Autodesk Inventor part; units mm, degrees
ref_plane "YZ Plane" through (0, 0, 0) normal (1, 0, 0) x (0, 1, 0)
ref_plane "XZ Plane" through (0, 0, 0) normal (0, 1, 0) x (-1, 0, 0)
ref_plane "XY Plane" through (0, 0, 0) normal (0, 0, 1) x (1, 0, 0)
sketch "Sketch1" plane through (0, 0, 0) normal (0, 0, 1) x (1, 0, 0)
  line L0 (0, 0) -> (0, 80)
  line L1 (0, 0) -> (25, 0)
  line L2 (25, 0) -> (25, 80)
  arc A0 (25, 80) -> (0, 80) centre (12.5, 58.3494) ccw
  dimension "d2" = 80
  dimension "d4" = 25
  dimension "d5" = 80
  dimension "d6" = 25
extrude "Extrusion1" add sketch "Sketch1" along normal blind 3
sketch "Sketch2" plane through (0, 0, 3) normal (0, 0, 1) x (1, 0, 0)
  circle A0 centre (12.5, 67.7859) radius 10
  point P0 (0, 0)
  dimension "d9" = 20
extrude "Extrusion2" cut sketch "Sketch2" against normal blind 3
sketch "Sketch3" plane through (0, 0, 0) normal (0, -1, 0) x (1, 0, 0)
  line L0 (25, 0) -> (0, 0)
  line L1 (25, 3) -> (0, 3)
  line L2 (0, 0) -> (25, 0)
  line L3 (25, 0) -> (25, 3)
  line L4 (25, 3) -> (0, 3)
  line L5 (0, 3) -> (0, 0)
extrude "Extrusion3" add sketch "Sketch3" along normal blind 50
sketch "Sketch4" plane through (0, -50, 0) normal (0, -1, 0) x (1, 0, 0)
  line L0 (0, 0) -> (0, 3)
  line L1 (25, 0) -> (25, 3)
  line L2 (0, 3) -> (25, 3)
  line L3 (25, 3) -> (25, 0)
  line L4 (25, 0) -> (0, 0)
  line L5 (0, 0) -> (0, 3)
sketch "Sketch5" plane through (0, 0, 3) normal (0, 0, 1) x (1, 0, 0)
  circle A0 centre (12.7766, 13.1416) radius 10
  point P0 (0, 0)
  dimension "d14" = 20
extrude "Extrusion4" cut sketch "Sketch5" against normal blind 50
sketch "Sketch6" plane through (0, 0, 3) normal (0, 0, 1) x (1, 0, 0)
  line L0 (31.6061, 27.9408) -> (-29.0129, 27.9408)
  line L1 (-29.0129, 27.9408) -> (-29.0129, 90.0456)
  line L2 (-29.0129, 90.0456) -> (31.6061, 90.0456)
  line L3 (31.6061, 90.0456) -> (31.6061, 27.9408)
  point P0 (0, 0)
extrude "Extrusion5" cut sketch "Sketch6" against normal blind 50
sketch "Sketch7" plane through (0, 0, 3) normal (0, 0, 1) x (1, 0, 0)
  point P0 (0, 0)
properties part number "roller support"
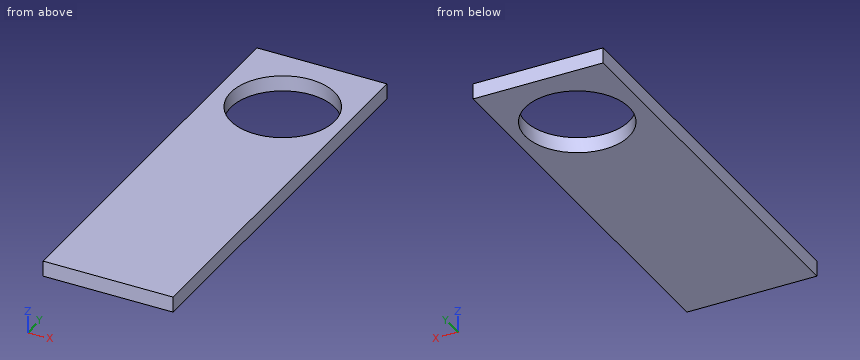
Input: part model. Units: mm. Frame: model coordinates. Coordinates: 2 decimals unless noted, no trailing zeros. Loops run counter-clockwise (first coordinate to the right, second up) from the corner with the lowest first, then second, coordinate; pieces in that order, holes last. Notation, with made-up numbers: (19, 16) -> (36, 16) arc R21 cw to (36, 47) -> close; hole circle Ø4 at (89.5, 68.5). An arc over 180 degrees is marked (long way). One line per item, written item: value.
(1) Cut plane A-A (x = 5.5). Output: boundary loops of the cut face in (y, z).
Answer below:
outline: (-50, 0) -> (6.28, 0) -> (6.28, 3) -> (-50, 3) -> close; (20, 0) -> (27.94, 0) -> (27.94, 3) -> (20, 3) -> close
(2) Ray query, line 1 along X through (y, z) = (18, 1); line 2 along Y through (x, z) = (16.5, 2.5); line 3 along Y through (x, z) = (11, 2.5). Return the intervals inside material, ascending.
Answer below:
line 1: x = 0 to 4.04, 21.52 to 25
line 2: y = -50 to 3.86, 22.42 to 27.94
line 3: y = -50 to 3.3, 22.98 to 27.94
(3) Cut plane C-C (z = 1.85). Output: boundary loops of the cut face in (x, y), then the cut area to 3 significant figures.
Answer below:
outline: (0, -50) -> (25, -50) -> (25, 27.94) -> (0, 27.94) -> close; hole circle Ø20 at (12.78, 13.14)
area: 1,630 mm2
(4) Pin query (flat end, axial travel): pin 1 Ø12 at (x, y) = (16.5, 6.5) entering from -Z. Return the tip coordinate at first contact, or that it passes through.
Answer below:
pin 1: stops at z = 0
(5) Cut plane B-B (y = 14.5). Output: boundary loops of the cut face in (x, z), then the cut area to 3 significant figures.
Answer below:
outline: (0, 0) -> (2.87, 0) -> (2.87, 3) -> (0, 3) -> close; (22.68, 0) -> (25, 0) -> (25, 3) -> (22.68, 3) -> close
area: 15.6 mm2
